Can you work these out from the model? Positions are in its coordinate system, mm. A direction names the side the tool comes from. Give positions to 0.01 mm unless a question says otherwise; leave off trailing zeros. Order: outer loops, then holes, each group sorted by start corner. A loop starts at its lowest first (then second) coordinate and runs counter-clockwise, first axis right, second up. Notation, with made-up numbers: M 79.5,-16 L 98.5,-16 A22 ccw 98.5,1 Z; hole C 61.25,77 d4. An arc over 180 degrees is marked long. Answer as a JSON object with one key per item and string values.
```python
from build123d import *

# Parameters (mm, degrees)
SKETCH1_W           = 68.58
SKETCH1_H           = 55.88
BOSS_EXTRUDE1_DEPTH = 3.81
SKETCH2_W           = 12.7
SKETCH2_H           = 10.16
BOSS_EXTRUDE2_DEPTH = 59.69
SKETCH6_W           = 12.7
SKETCH6_H           = 20.32
BOSS_EXTRUDE3_DEPTH = 35.56
CUT_EXTRUDE1_REACH  = 108.718
SKETCH4_R           = 11.303
SKETCH7_W           = 68.58
SKETCH7_H           = 55.88
SKETCH7_W_2         = 43.18
SKETCH7_H_2         = 22.86
BOSS_EXTRUDE4_DEPTH = 2.54
SKETCH8_R           = 3.429
SKETCH8_R_2         = 7.493
CUT_EXTRUDE2_DEPTH  = 2.54
SKETCH9_W           = 68.58
SKETCH9_H           = 22.987
BOSS_EXTRUDE5_DEPTH = 2.54
CUT_EXTRUDE3_REACH  = 110.159
SKETCH10_W          = 12.446
SKETCH10_H          = 3.048
SKETCH11_W          = 15.367
SKETCH11_H          = 22.987
BOSS_EXTRUDE6_DEPTH = 12.7
BOSS_EXTRUDE7_DEPTH = 22.86
CUT_EXTRUDE5_START  = -43.18
SKETCH14_R          = 12.7
CUT_EXTRUDE5_DEPTH  = 43.18
CUT_EXTRUDE6_REACH  = 102.587
SKETCH13_R          = 10.287
SKETCH15_R          = 31.640904619
CUT_EXTRUDE7_DEPTH  = 7.62


with BuildPart() as part:
    # Sketch1 → Boss-Extrude1 (new body)
    with BuildSketch(Plane.XY):
        with Locations((34.29, 27.94)):
            Rectangle(SKETCH1_W, SKETCH1_H)
    extrude(amount=BOSS_EXTRUDE1_DEPTH)

    # Sketch2 → Boss-Extrude2 (add)
    with BuildSketch(Plane(origin=(0, 0, 0), x_dir=(-1, 0, 0), z_dir=(0, 0, -1))):
        with Locations((-6.35, 50.8)):
            Rectangle(SKETCH2_W, SKETCH2_H)
        with Locations((-62.23, 50.8)):
            Rectangle(SKETCH2_W, SKETCH2_H)
        with Locations((-6.35, 5.08)):
            Rectangle(SKETCH2_W, SKETCH2_H)
        with Locations((-62.23, 5.08)):
            Rectangle(SKETCH2_W, SKETCH2_H)
    extrude(amount=BOSS_EXTRUDE2_DEPTH)

    # Sketch6 → Boss-Extrude3 (add)
    with BuildSketch(Plane(origin=(0, 10.16, 0), x_dir=(1, 0, 0), z_dir=(0, 1, 0))):
        with Locations((62.23, 49.53)):
            Rectangle(SKETCH6_W, SKETCH6_H)
        with Locations((6.35, 49.53)):
            Rectangle(SKETCH6_W, SKETCH6_H)
    extrude(amount=BOSS_EXTRUDE3_DEPTH)

    # Sketch4 → Cut-Extrude1 (cut, up to next)
    with BuildSketch(Plane(origin=(68.58, 0, 0), x_dir=(0, 0, -1), z_dir=(1, 0, 0)), mode=Mode.PRIVATE) as cut_extrude1_sk1:
        with Locations((49.53, 27.94)):
            Circle(SKETCH4_R)
    cut_extrude1_tool1 = extrude(cut_extrude1_sk1.sketch, amount=-CUT_EXTRUDE1_REACH, mode=Mode.PRIVATE) & part.part
    add(cut_extrude1_tool1.solids().sort_by_distance((68.58, 27.94, -49.53))[0], mode=Mode.SUBTRACT)

    # Sketch7 → Boss-Extrude4 (add)
    with BuildSketch(Plane(origin=(0, 0, -7.62), x_dir=(-1, 0, 0), z_dir=(0, 0, -1))):
        with Locations((-34.29, 27.94)):
            Rectangle(SKETCH7_W, SKETCH7_H)
        with Locations((-34.29, -11.43)):
            Rectangle(SKETCH7_W_2, SKETCH7_H_2)
    extrude(amount=BOSS_EXTRUDE4_DEPTH)

    # Sketch8 → Cut-Extrude2 (cut)
    with BuildSketch(Plane(origin=(0, 0, -10.16), x_dir=(-1, 0, 0), z_dir=(0, 0, -1))):
        with Locations((-34.29, -10.16)):
            Circle(SKETCH8_R)
        with Locations((-34.29, 27.94)):
            Circle(SKETCH8_R_2)
    extrude(amount=-CUT_EXTRUDE2_DEPTH, mode=Mode.SUBTRACT)

    # Sketch9 → Boss-Extrude5 (add)
    with BuildSketch(Plane(origin=(0, 0, -59.69), x_dir=(-1, 0, 0), z_dir=(0, 0, -1))):
        with Locations((-34.29, 11.4935)):
            Rectangle(SKETCH9_W, SKETCH9_H)
    extrude(amount=BOSS_EXTRUDE5_DEPTH)

    # Sketch10 → Cut-Extrude3 (cut, up to next)
    with BuildSketch(Plane.XZ, mode=Mode.PRIVATE) as cut_extrude3_sk1:
        with Locations((34.29, -59.69)):
            Rectangle(SKETCH10_W, SKETCH10_H)
    cut_extrude3_tool1 = extrude(cut_extrude3_sk1.sketch, amount=-CUT_EXTRUDE3_REACH, mode=Mode.PRIVATE) & part.part
    add(cut_extrude3_tool1.solids().sort_by_distance((34.29, 0, -59.69))[0], mode=Mode.SUBTRACT)

    # Sketch11 → Boss-Extrude6 (add)
    with BuildSketch(Plane.XY.offset(-59.69)):
        with Locations((20.3835, 11.4935)):
            Rectangle(SKETCH11_W, SKETCH11_H)
        with Locations((48.1965, 11.4935)):
            Rectangle(SKETCH11_W, SKETCH11_H)
    extrude(amount=BOSS_EXTRUDE6_DEPTH)

    # Sketch12 → Boss-Extrude7 (add)
    with BuildSketch(Plane.XZ):
        Polygon((12.7, -10.16), (0, -10.16), (0, 3.81), (68.58, 3.81), (68.58, -10.16), (55.88, -10.16), (55.88, 0), (12.7, 0), align=None)
    extrude(amount=BOSS_EXTRUDE7_DEPTH)

    # Sketch14 → Cut-Extrude5 (cut)
    with BuildSketch(Plane(origin=(55.88, 0, 0), x_dir=(0, 0, -1), z_dir=(1, 0, 0)).offset(CUT_EXTRUDE5_START)):
        with Locations((49.53, 27.94)):
            Circle(SKETCH14_R)
    extrude(amount=CUT_EXTRUDE5_DEPTH, mode=Mode.SUBTRACT)

    # Sketch13 → Cut-Extrude6 (cut, up to next)
    with BuildSketch(Plane(origin=(12.7, 0, 0), x_dir=(0, 0, -1), z_dir=(1, 0, 0)), mode=Mode.PRIVATE) as cut_extrude6_sk1:
        with Locations((49.53, 27.94)):
            Circle(SKETCH13_R)
    cut_extrude6_tool1 = extrude(cut_extrude6_sk1.sketch, amount=-CUT_EXTRUDE6_REACH, mode=Mode.PRIVATE) & part.part
    add(cut_extrude6_tool1.solids().sort_by_distance((12.7, 27.94, -49.53))[0], mode=Mode.SUBTRACT)

    # Sketch15 → Cut-Extrude7 (cut)
    with BuildSketch(Plane(origin=(0, 0, 0), x_dir=(-1, 0, 0), z_dir=(0, 0, -1))):
        with Locations((-34.29, 27.94)):
            Circle(SKETCH15_R)
    extrude(amount=CUT_EXTRUDE7_DEPTH, mode=Mode.SUBTRACT)


solid = part.part
```
1) I'm going to push flat-ended pins straight in: pin 1 Ø15.5 at (x, z) = (50, -33.5) entering from -Y; pin 2 Ø24 at (x, y) = (34.29, 27.94) entering from -Z; pin 3 Ø6 at (x, y) = (34.29, -10.16) entering from -Z; pin 4 Ø5 at (y, z) = (13.5, -21.5) entering from -X. Where does each tip first touch, or does it pass through?
Results found:
{"pin 1": "stops at y = 0", "pin 2": "stops at z = -62.23", "pin 3": "stops at z = 0", "pin 4": "passes through"}
2) I want a section at D-D on x = 34.29. Count the separate pieces of the cut face and the enclosed holes in it, and give its area (3 significant figures).
Results found:
{"separate pieces": "5", "enclosed holes": "0", "area": "468 mm²"}
3) For faces 1 (the face through (10.23, 48.49, -3.76)), 2 (the face through (12.7, 48, -40)), 3 (the face through (62, 16, -39.37)), 4 (the face through (40.513, 9, -54)), which set-ups out of +Z, -Z, +X, -X, +Y, -Y let a thin tool reach every point of the face, with its end or its side?
Results found:
{"face 1": "none", "face 2": "-Z, +Y", "face 3": "+X, -X", "face 4": "+Y, -Y"}
4) I need wall thicknesses on L1, parallel to Z at x = 42, y = 13.5; L2, parallel to Y at x = 34.29, z = -8.15; L3, parallel to Y at x = 34, z = -8. Which ranges of each line are inside material? Lowest first, please.
Results found:
{"L1": "z = -62.23 to -46.99, -10.16 to -7.62, 0 to 3.81", "L2": "y = -22.86 to -13.59, -6.73 to 20.45, 35.43 to 55.88", "L3": "y = -22.86 to -13.58, -6.74 to 20.45, 35.43 to 55.88"}
5) I want a section at C-C on y = 27.94. Write out the boundary of the cut face in (x, z).
Results found:
{"outline": "M 0,-10.16 L 26.8,-10.16 L 26.8,-7.62 L 0,-7.62 Z; M 0,0 L 68.58,0 L 68.58,3.81 L 0,3.81 Z; M 41.78,-10.16 L 68.58,-10.16 L 68.58,-7.62 L 41.78,-7.62 Z"}
6) I want a section at A-A on z = -33. Write out the boundary of the cut face in (x, y), and give its area (3 significant figures).
Results found:
{"outline": "M 0,0 L 12.7,0 L 12.7,10.16 L 0,10.16 Z; M 0,45.72 L 12.7,45.72 L 12.7,55.88 L 0,55.88 Z; M 55.88,0 L 68.58,0 L 68.58,10.16 L 55.88,10.16 Z; M 55.88,45.72 L 68.58,45.72 L 68.58,55.88 L 55.88,55.88 Z", "area": "516 mm²"}
7) Thinking about a two-plate mould opening in Z: for faces 5 (the face through (68.58, 7, -21)), 6 (the face through (34, 17, 3.81)), 7 (the face through (58.29, 48.56, -3.76)), which applies, pulls with the +Z half, pulls with the -Z half, needs draft (parallel to the pull), parting line crosses it, or undercut?
Results found:
{"face 5": "needs draft", "face 6": "pulls with the +Z half", "face 7": "undercut"}
8) I want a section at B-B on x = 18. Write out the boundary of the cut face in (y, z).
Results found:
{"outline": "M -22.86,-10.16 L 55.88,-10.16 L 55.88,-7.62 L -22.86,-7.62 Z; M -22.86,0 L 55.88,0 L 55.88,3.81 L -22.86,3.81 Z; M 0,-62.23 L 22.99,-62.23 L 22.99,-61.22 A12.7 cw 15.5,-46.99 L 0,-46.99 Z"}
